Read the model definition and answer for the solid it produces. Units are mm, in the model's axes. A direction names the side the tool comes from. Coordinates: 2 decimals unless noted, no trailing zeros. Order: outer loops, then holes, each group sorted by start corner. A loop starts at its lowest first (then second) coordinate and runs counter-clockwise, first axis right, second up. Notation, with made-up numbers: M 1,30.5 L 35,30.5 A15 ccw 35,56.5 Z; hole C 60.25,-34.5 d5. An arc over 180 degrees is marked long. Put each result on its own line as item: value.
from build123d import *

# Parameters (mm, degrees)
F0_W     = 25.4
F0_H     = 25.4
F0_W_2   = 22.225
F0_H_2   = 22.225
F1_DEPTH = 152.4
F3_DEPTH = 25.4


with BuildPart() as f1:
    # F0 (on Top) → F1 (new body)
    with BuildSketch(Plane.XY):
        Rectangle(F0_W, F0_H)
        Rectangle(F0_W_2, F0_H_2, mode=Mode.SUBTRACT)
    extrude(amount=F1_DEPTH)

    # F2 (on face) → F3 (cut, through all)
    with BuildSketch(Plane.YZ.offset(12.7)):
        Polygon((12.7, 152.4), (-12.7, 152.4), (12.7, 127), align=None)
        Polygon((12.7, 25.4), (-12.7, 0), (12.7, 0), align=None)
    extrude(amount=-F3_DEPTH, mode=Mode.SUBTRACT)


solid = f1.part
Q1. Find section D-D on z = 11. Write down the section's boundary in (x, y).
Answers below:
outline: M -12.7,-12.7 L 12.7,-12.7 L 12.7,-1.7 L 11.11,-1.7 L 11.11,-11.11 L -11.11,-11.11 L -11.11,-1.7 L -12.7,-1.7 Z
Q2. A tool of negligible diameter and unlimited length cuts with its end or side. For faces 1 (the face through (0, -11.112, 75)), 2 (the face through (-12.7, 0, 75)), from which of +Z, -Z, +X, -X, +Y, -Y can it reach the whole face along a straight path? Write none if from no direction.
Answers below:
face 1: +Z, -Z
face 2: +Z, -Z, -X, +Y, -Y
Q3. Find section C-C on z = 40. Write down the section's boundary in (x, y), plus the area to 3 significant figures.
Answers below:
outline: M -12.7,-12.7 L 12.7,-12.7 L 12.7,12.7 L -12.7,12.7 Z; hole M -11.11,-11.11 L 11.11,-11.11 L 11.11,11.11 L -11.11,11.11 Z
area: 151 mm^2
Q4. Find section A-A on y = -5. Write down the section's boundary in (x, z), plus the area to 3 significant figures.
Answers below:
outline: M -12.7,7.7 L -11.11,7.7 L -11.11,144.7 L -12.7,144.7 Z; M 11.11,7.7 L 12.7,7.7 L 12.7,144.7 L 11.11,144.7 Z
area: 435 mm^2
Q5. For a pull along X with two mould halves and no side action, classify faces 3 (the face through (0, -12.7, 75)), 4 (the face through (12.7, 0, 75)), 5 (the face through (-11.112, 0, 75)) as +X half, -X half, draft (parallel to the pull), parting line (faces both ways), or undercut.
Answers below:
face 3: draft
face 4: +X half
face 5: undercut
Q6. Given pin 1 (12 mm diameter, centred on x = -0.5, y = 9, fed in from +Z), flat-ended and moving along its own axis, determine where the tip first touches the part or whether it passes through.
Answers below:
pin 1: stops at z = 128.59
Q7. Consider line 1 along X through (y, z) = (-10.25, 130); line 2 along Y through (x, z) = (-7.5, 11.5). Determine where each line is inside the solid, lowest interval first.
Answers below:
line 1: x = -12.7 to -11.11, 11.11 to 12.7
line 2: y = -12.7 to -11.11
Q8. Find section B-B on x = -8.25. Write down the section's boundary in (y, z), plus the area to 3 significant figures.
Answers below:
outline: M -12.7,0 L -11.11,1.59 L -11.11,150.81 L -12.7,152.4 Z; M 11.11,23.81 L 12.7,25.4 L 12.7,127 L 11.11,128.59 Z
area: 403 mm^2
